Can you work these out from the drawing? Everything is in mm from the part's minimum corner. A direction names the side the tool comes from. Round coordinates to 2 decimals unless told otherwise and drop trailing zeros. Write each loop counter-clockwise with the first axis right and the second up, starting at its lowest first coordinate (ties: lowest second). Pieces come first, ordered by that corner, then holes.
Q1. For the marked faces 1 and 2, which set-ups out of +Z, -Z, +X, -X, +Y, -Y let a thin tool reach every point of the face, with its end or its side?
Q2. If we section it at B-B (y = 25): Please give me the cut outline in (x, z).
Q3. We'd pull the mould along X, two halves only. Please class the marked faces 3, 4, 5 and 6: +X half, -X half, draft (parallel to the pull), parting line (faces both ways), or undercut.
Q4. I'm going to push flat-ended pins straight in: pin 1 Ø1 at (y, z) = (40, 5) entering from -X (1 decimal); pin 2 Ø6 at (y, z) = (38.5, 7) entering from -X (1 decimal); pin 3 Ø1.5 at (x, z) = (44.5, 3) entering from +Y (1 decimal). Where does each tip first touch, or does it pass through?
Q5. If we section it at D-D (y = 10): Please give me the cut outline in (x, z) (1 decimal), plus the area to 3 significant figures.
Q6. Please list where these lines run through material, in increasing order: line 1 along Y through (x, z) = (25, 8.9); line 2 along Y through (x, z) = (25, 1.35); line 3 along Z through (x, y) = (38, 37).
Q7. If we section it at A-A (z = 6.75): Please give me the cut outline in (x, y) (1 decimal).
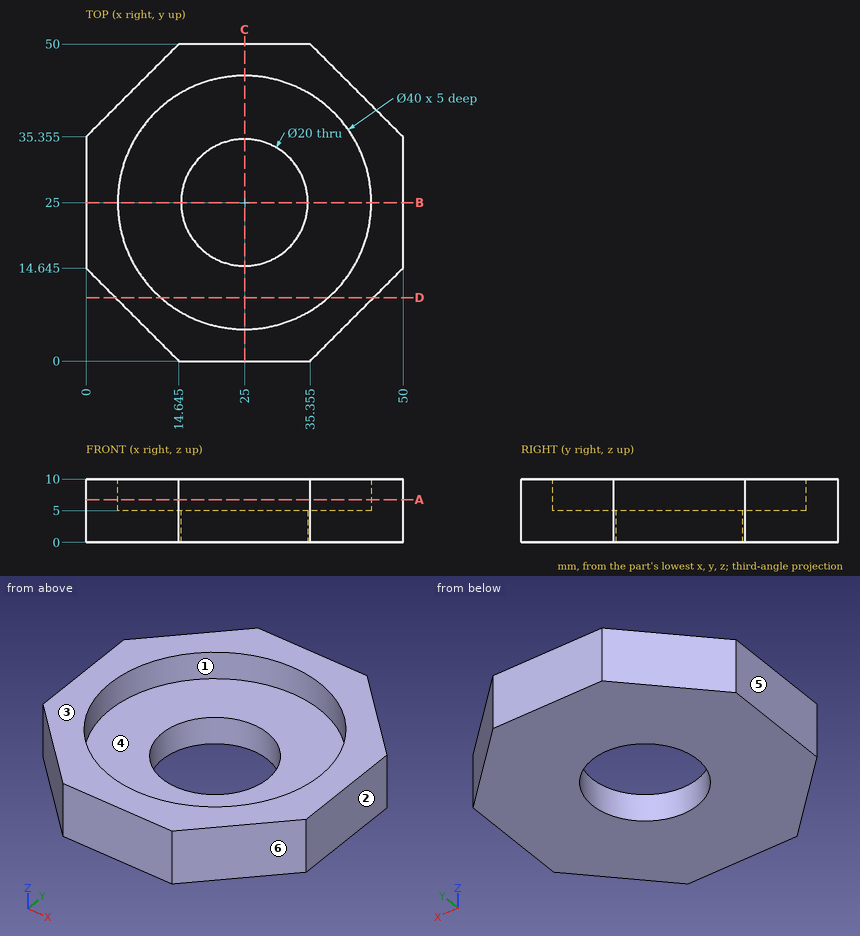
A:
1. face 1: +Z
1. face 2: +Z, -Z, +X, +Y, -Y
2. outline: (0, 0) - (15, 0) - (15, 5) - (5, 5) - (5, 10) - (0, 10) - close; (35, 0) - (50, 0) - (50, 10) - (45, 10) - (45, 5) - (35, 5) - close
3. face 3: draft
3. face 4: undercut
3. face 5: -X half
3. face 6: +X half
4. pin 1: stops at x = 4.1
4. pin 2: stops at x = 0.1
4. pin 3: stops at y = 41.6
5. outline: (4.6, 0) - (45.4, 0) - (45.4, 10) - (38.2, 10) - (38.2, 5) - (11.8, 5) - (11.8, 10) - (4.6, 10) - close
5. area: 275 mm2
6. line 1: y = 0 to 5, 45 to 50
6. line 2: y = 0 to 15, 35 to 50
6. line 3: z = 0 to 5
7. outline: (0, 14.6) - (14.6, 0) - (35.4, 0) - (50, 14.6) - (50, 35.4) - (35.4, 50) - (14.6, 50) - (0, 35.4) - close; hole circle Ø40 at (25, 25)
